from build123d import *

# Parameters (mm, degrees)
SKETCH_W        = 35
SKETCH_H        = 17.5
SKETCH_R        = 2.65
SKETCH_W_2      = 13
SKETCH_H_2      = 5
PAD_DEPTH       = 30
SKETCH001_R     = 3.55
POCKET_DEPTH    = 17.501
SKETCH002_W     = 13
SKETCH002_H     = 7.5
POCKET001_DEPTH = 5


with BuildPart() as part:
    # Sketch → Pad (new body)
    with BuildSketch(Plane.XZ):
        Rectangle(SKETCH_W, SKETCH_H)
        with Locations((-12, 0)):
            Circle(SKETCH_R, mode=Mode.SUBTRACT)
        with Locations((12, 0)):
            Circle(SKETCH_R, mode=Mode.SUBTRACT)
        with Locations((0, -3.25)):
            Rectangle(SKETCH_W_2, SKETCH_H_2, mode=Mode.SUBTRACT)
    extrude(amount=PAD_DEPTH)

    # Sketch001 (on DatumPlane) → Pocket (cut, through all)
    with BuildSketch(Plane(origin=(0, 0, 8.75), x_dir=(-1, 0, 0), z_dir=(0, 0, 1))):
        with Locations((0, 15)):
            Circle(SKETCH001_R)
    extrude(amount=-POCKET_DEPTH, mode=Mode.SUBTRACT)

    # Sketch002 → Pocket001 (cut)
    with BuildSketch(Plane(origin=(0, 0, -7.5), x_dir=(1, 0, 0), z_dir=(0, 0, -1))):
        with Locations((0, 15)):
            Rectangle(SKETCH002_W, SKETCH002_H)
    extrude(amount=-POCKET001_DEPTH, mode=Mode.SUBTRACT)


solid = part.part
Geometry check sheet. Reference: the model listing, model coordinates, mm. A direction names the side the tool comes from. Coordinates: 2 decimals unless noted, no trailing zeros. Order: outer loops, then holes, each group sorted by start corner. A loop starts at its lowest first (then second) coordinate and runs counter-clockwise, first axis right, second up. Notation, with made-up numbers: (50, 34) -> (109, 34) arc R24 cw to (109, 67) -> close; hole circle Ø11 at (-39, 37). An arc over 180 degrees is marked (long way). Use a Markdown table: item, result. Add a question column.
1. Mould release check, pull along X, two halves, no side actions. Record for faces 4 (the face through (-17.5, -15, 0)), 5 (the face through (-2, -11, -0.75)), 6 (the face through (0, -30, 0)), 7 (the face through (17.5, -15, 0)): pulls with the +X half, pulls with the -X half, needs draft (parallel to the pull), parting line crosses it, or undercut.
2. Cross-section at B-B (x = -12). Enter the section's corners in (y, z).
3. Cross-section at A-A (z = 0). Enter the section's corners in (x, y).
4. Cross-section at D-D (y = -15). Enter the section's corners in (x, z), and give its area (3 significant figures).
5. Cross-section at C-C (z = -4). Enter the section's corners in (x, y), and give its area (3 significant figures).
6. Set-up check for faces 1 (the face through (0, 0, 0)), 2 (the face through (0, -11.25, -7)), 3 (the face through (0, -6, -5.75)): record each of +Z, -Z, +X, -X, +Y, -Y from which the full face is reachable in a straight line by a thin tool's end or side.
7. Material ranges on L1, parallel to Z at x = -12, y = -23; L2, parallel to X at y = -20, z = -1; L3, parallel to Z at x = 4, y = -21, recorded low to high.
Filled sheet:
| question | item | result |
|---|---|---|
| 1 | face 4 | pulls with the -X half |
| 1 | face 5 | undercut |
| 1 | face 6 | needs draft |
| 1 | face 7 | pulls with the +X half |
| 2 | outline | (-30, -8.75) -> (0, -8.75) -> (0, -2.65) -> (-30, -2.65) -> close; (-30, 2.65) -> (0, 2.65) -> (0, 8.75) -> (-30, 8.75) -> close |
| 3 | outline | (-17.5, -30) -> (-14.65, -30) -> (-14.65, 0) -> (-17.5, 0) -> close; (-9.35, -30) -> (9.35, -30) -> (9.35, 0) -> (-9.35, 0) -> close; (14.65, -30) -> (17.5, -30) -> (17.5, 0) -> (14.65, 0) -> close; hole circle Ø7.1 at (0, -15) |
| 4 | outline | (-17.5, -8.75) -> (-3.55, -8.75) -> (-3.55, -7.5) -> (-6.5, -7.5) -> (-6.5, -0.75) -> (-3.55, -0.75) -> (-3.55, 8.75) -> (-17.5, 8.75) -> close; (3.55, -8.75) -> (17.5, -8.75) -> (17.5, 8.75) -> (3.55, 8.75) -> (3.55, -0.75) -> (6.5, -0.75) -> (6.5, -7.5) -> (3.55, -7.5) -> close; hole circle Ø5.3 at (-12, 0); hole circle Ø5.3 at (12, 0) |
| 4 | area | 404 mm2 |
| 5 | outline | (-17.5, -30) -> (-6.5, -30) -> (-6.5, 0) -> (-17.5, 0) -> close; (6.5, -30) -> (17.5, -30) -> (17.5, 0) -> (6.5, 0) -> close |
| 5 | area | 660 mm2 |
| 6 | face 1 | +Z, -Z, +X, -X, +Y |
| 6 | face 2 | none |
| 6 | face 3 | +Y, -Y |
| 7 | L1 | -8.75 to -2.65, 2.65 to 8.75 |
| 7 | L2 | -17.5 to -14.45, -9.55 to -6.5, 6.5 to 9.55, 14.45 to 17.5 |
| 7 | L3 | -8.75 to -5.75, -0.75 to 8.75 |
